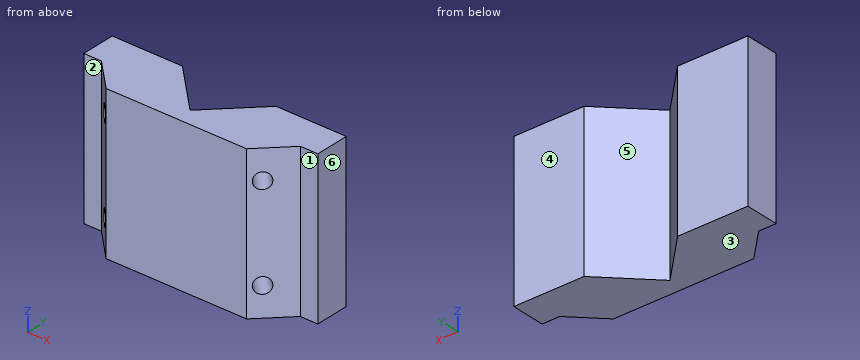
from build123d import *

# Parameters (mm, degrees)
BOSS_EXTRUDE1_DEPTH            = 32.5
TALADRO_ROSCADO_M86_AT_2_COUNT = 2
TALADRO_ROSCADO_M86_AT_2_PITCH = 40


with BuildPart() as part:
    # Sketch1 → Boss-Extrude1 (new body, symmetric)
    with BuildSketch(Plane.XY):
        Polygon((-30, 0), (30, 0), (42.5, 12.5), (50, 12.5), (50, 27), (20, 27), (0, 7), (-20, 27), (-50, 27), (-50, 12.5), (-42.5, 12.5), align=None)
    extrude(amount=BOSS_EXTRUDE1_DEPTH, both=True)

    # Croquis12 → Taladro roscado M86 (revolve, cut)
    with BuildSketch(Plane(origin=(33.725048023, 3.725048023, 20), x_dir=(0.707106781, 0.707106781, 0), z_dir=(0, 0, 1))):
        Polygon((0, 0), (0, 22.042926105), (3.4, 20), (3.4, 0), align=None)
    taladro_roscado_m86 = revolve(axis=Axis((38.215176084, -0.765080037, 20), (-0.707106781, 0.707106781, 0)), mode=Mode.SUBTRACT)

    # Taladro roscado M86 at 2: Taladro roscado M86 ×2
    with Locations(*[(0, 0, -i * TALADRO_ROSCADO_M86_AT_2_PITCH) for i in range(1, TALADRO_ROSCADO_M86_AT_2_COUNT)]):
        add(taladro_roscado_m86, mode=Mode.SUBTRACT)

    # Simetría3: Taladro roscado M86 across plane
    add(taladro_roscado_m86.mirror(Plane(origin=(0, 0, 0), x_dir=(0, 0, 1), z_dir=(1, 0, 0))), mode=Mode.SUBTRACT)

    # Simetría3 copy 1 sketch → Simetría3 copy 1 (revolve, cut)
    with BuildSketch(Plane(origin=(-33.725048023, 3.725048023, -20), x_dir=(-0.707106781, 0.707106781, 0), z_dir=(0, 0, 1))):
        Polygon((0, 0), (0, -22.042926105), (3.4, -20), (3.4, 0), align=None)
    revolve(axis=Axis((-38.215176084, -0.765080037, -20), (-0.707106781, -0.707106781, 0)), mode=Mode.SUBTRACT)


solid = part.part
Work out the finished part from the listing and answer in its coordinate system (mm). Face numbers are marked on the shaded views. A direction names the side the tool comes from. Give positions to 0.01 mm unless a question says otherwise; leave off trailing zeros. Write each loop counter-clockwise with the first axis right and the second up, starting at its lowest first coordinate (ties: lowest second). Pieces come first, ordered by that corner, then holes. Notation, with made-up numbers: (50.25, 62.25) - (100.25, 62.25) arc R24 ccw to (100.25, 75.25) - close; hole circle Ø3 at (14, -9). An arc over 180 degrees is marked (long way). One line per item, written item: value. Start each with the question number.
1. Find section D-D (y = 10.75). State how many separate pieces and enclosed holes the cut face has, then the cut area to 3 significant figures.
2. For the marked faces 1, 2 and 3, determine the directions among +Z, -Z, +X, -X, +Y, -Y from which every point of the face is accessible in a straight line to the end or side of a thin tool.
3. Consider probe 1 along X at (y, z) = (15.75, 20); probe 2 along X at (y, z) = (16.5, 22); probe 3 along X at (y, z) = (17.5, -23.5). Determine where each line is inside the solid, lowest interval first.
4. Find section B-B (z = 10.5). Write down the section's boundary in (x, y), then the cut area to 3 significant figures.
5. Find section C-C (x = 7). Write down the section's boundary in (y, z).
6. Find section A-A (y = 23.5). Write down the section's boundary in (x, z).
7. Given pin 1 (4 mm diameter, centred on x = 31, z = -19.5, fed in from -Y); pin 2 (10 mm diameter, centred on y = 4, z = -21, fed in from +X); pin 3 (8 mm diameter, centred on x = 47, z = -0.5, fed in from -Y), each flat-ended and moving along its own axis, determine where each tip first touches the part or whether it passes through.
8. For a pull along X with two mould halves and no side action, classify the marked faces 4, 5 and 6 as +X half, -X half, draft (parallel to the pull), parting line (faces both ways), or undercut.
Geometry results:
1. separate pieces: 2
1. enclosed holes: 4
1. area: 4,600 mm2
2. face 1: +Z, -Z, +X, -Y
2. face 2: +Z, -Z, -X, -Y
2. face 3: -Z, +X, -X, +Y, -Y
3. probe 1: -50 to -26.51, -17.25 to -8.75, 8.75 to 17.25, 26.51 to 50
3. probe 2: -50 to -24.84, -17.85 to -9.5, 9.5 to 17.85, 24.84 to 50
3. probe 3: -50 to -10.5, 10.5 to 50
4. outline: (-50, 12.5) - (-42.5, 12.5) - (-30, 0) - (30, 0) - (42.5, 12.5) - (50, 12.5) - (50, 27) - (20, 27) - (0, 7) - (-20, 27) - (-50, 27) - close
4. area: 1,960 mm2
5. outline: (0, -32.5) - (14, -32.5) - (14, 32.5) - (0, 32.5) - close
6. outline: (-50, -32.5) - (-16.5, -32.5) - (-16.5, 32.5) - (-50, 32.5) - close; (16.5, -32.5) - (50, -32.5) - (50, 32.5) - (16.5, 32.5) - close
7. pin 1: y = 0
7. pin 2: x = 39
7. pin 3: y = 12.5
8. face 4: draft
8. face 5: undercut
8. face 6: +X half
